Can you work these out from the model? Positions are in its coordinate system, mm. Face numbers are marked on the shaded views. A direction names the side the tool comes from. Coordinates: 2 decimals unless noted, no trailing zeros. Loops run counter-clockwise (first coordinate to the right, second up) from the corner with the lowest first, then second, coordinate; pieces in that order, holes last. Notation, with made-up numbers: (33, 51.25) - (82, 51.25) arc R9 ccw to (82, 57.25) - close; hole circle Ø9 at (8.25, -2.5). An arc over 180 degrees is marked (long way). Put each result on its own line as item: value. Start each with the question number.
from build123d import *

# Parameters (mm, degrees)
F2_W = 10
F2_H = 3
F5_D = 3.3
F7_D = 2.5


with BuildPart() as f3:
    # F3: sweep along a path in F0
    with BuildLine(Plane.YZ) as f3_path:
        Line((20, 0), (5, 0))
        ThreePointArc((5, 0), (1.4644660941, 1.4644660941), (0, 5))
        Line((0, 5), (0, 20))
    # F2 (on line) → F3 (sweep)
    with BuildSketch(Plane.XZ.offset(-20)):
        with Locations((-5, 1.5)):
            Rectangle(F2_W, F2_H)
    sweep(path=f3_path.line)

    # F5 (through all)
    with Locations(Plane.XY.offset(3)):
        with Locations((-5, 12.5)):
            Hole(F5_D / 2)

    # F7 (through all)
    with Locations(Plane(origin=(0, 3, 0), x_dir=(-1, 0, 0), z_dir=(0, 1, 0))):
        with Locations((5, 12.5)):
            Hole(F7_D / 2)


solid = f3.part
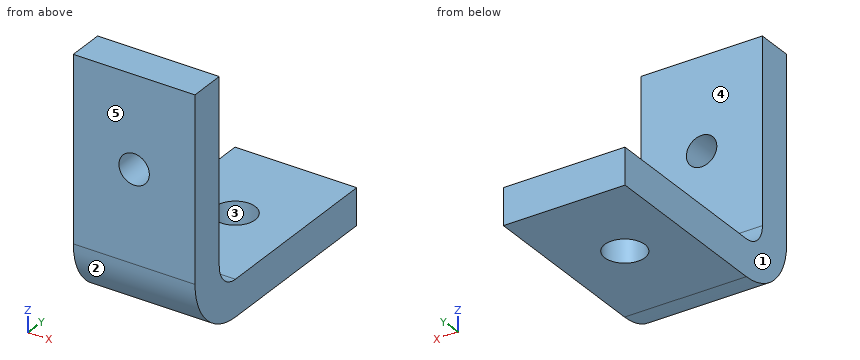
Q1. I want a section at B-B on y = 12.5. List the corners of the cut face in (x, z) for me, and give its area (3 significant figures).
Q2. On a 3-axis mill with a long thin cutter (end or side, diameter ignored), from which of +Z, -Z, +X, -X, +Y, -Y can I reach the whole of each face in a straight line? I mean the marked faces 4 and 5. Say none if no direction works.
Q3. I want a section at A-A on x = -5. List the corners of the cut face in (y, z) for me, and give its area (3 significant figures).
Q4. Please list where these lines run through material, in increasing order: line 1 along Y through (x, z) = (-4, 13.5); line 2 along Y through (x, z) = (-5, 1.15). Write a range as [from, to].
Q5. I want a section at C-C on z = 12.5. List the corners of the cut face in (x, y) for me.
Q6. I want a section at D-D on x = -2. List the corners of the cut face in (y, z) for me, and give its area (3 significant figures).
Q7. Will these pins go through, and if not, where does the flat tip stop? pin 1 (5 mm diameter, centred on x = -3.5, z = 11.5, fed in from +Y); pin 2 (3 mm diameter, centred on x = -5, z = 5, fed in from -Y); pin 3 (5 mm diameter, centred on x = -6, y = 16, fed in from +Z); pin 4 (3 mm diameter, centred on y = 17.5, z = 6, fed in from -X).
Q8. We'd pull the mould along X, two halves only. Please class the marked faces 1, 2 and 3: released by +X, released by -X, zero draft, split by the parting line, or undercut.
Calculated:
1. outline: (-10, 0) - (-6.65, 0) - (-6.65, 3) - (-10, 3) - close; (-3.35, 0) - (0, 0) - (0, 3) - (-3.35, 3) - close
1. area: 20.1 mm2
2. face 4: +Z, +X, -X, +Y
2. face 5: +Z, -Z, +X, -X, -Y
3. outline: (0, 5) arc R5 ccw to (5, 0) - (10.85, 0) - (10.85, 3) - (5, 3) arc R2 cw to (3, 5) - (3, 11.25) - (0, 11.25) - close; (0, 13.75) - (3, 13.75) - (3, 20) - (0, 20) - close; (14.15, 0) - (20, 0) - (20, 3) - (14.15, 3) - close
3. area: 89.1 mm2
4. line 1: [0, 3]
4. line 2: [1.81, 10.85], [14.15, 20]
5. outline: (-10, 0) - (-6.25, 0) - (-6.25, 3) - (-10, 3) - close; (-3.75, 0) - (0, 0) - (0, 3) - (-3.75, 3) - close
6. outline: (0, 5) arc R5 ccw to (5, 0) - (20, 0) - (20, 3) - (5, 3) arc R2 cw to (3, 5) - (3, 20) - (0, 20) - close
6. area: 106 mm2
7. pin 1: y = 3
7. pin 2: y = 0
7. pin 3: z = 3
7. pin 4: through
8. face 1: released by -X
8. face 2: zero draft
8. face 3: undercut
